Read the model definition and answer for the solid it produces. Units are mm, in the model's axes. A direction names the side the tool comes from. Round coordinates to 2 decimals unless told otherwise and drop trailing zeros. Order: outer loops, then holes, each group sorted by start corner. A loop starts at its lowest first (then second) coordinate and runs counter-clockwise, first axis right, second up. Notation, with made-up numbers: (2.5, 1) -> (14.5, 1) arc R22 cw to (14.5, 18) -> close; hole circle Ø8 at (18.25, -21). An arc over 180 degrees is marked (long way). Use a Markdown table: item, result. Add a question column.
1. Consider L1, parallel to X at y = -39.5, z = 6.25; L2, parallel to X at y = -26, z = 8.75; L3, parallel to X at y = -31.5, z = 3.5. Determine where each line is inside the solid, lowest interval first. Write a range as [from, to].
2. For faces 4 (the face through (-5, -26, 10)), 5 (the face through (-4, -46.502, 2)), 6 (the face through (66.314, -41.485, 6.302)), determine the directions among +Z, -Z, +X, -X, +Y, -Y from which every point of the face is accessible in a straight line to the end or side of a thin tool.
3. Given pin 1 (3 mm diameter, centred on y = -35, z = 4.5, fed in from -X); pin 2 (2 mm diameter, centred on x = 65.5, y = -39.5, fed in from +Z); pin 3 (5 mm diameter, centred on y = -18, z = 1.5, fed in from +X), each flat-ended and moving along its own axis, determine where each tip first touches the part or whether it passes through.
4. The mould has two halves that part along Y. Classify faces 1 (the face through (102.314, -30.797, 8.574)), 2 (the face through (-4, -26, 4)), 3 (the face through (-5.329, 1.994, 8.574)): +Y half, -Y half, draft (parallel to the pull), parting line (faces both ways), or undercut.
5. Section B-B, the plane z = 8 is taken. Give the vertices of the cut face in (x, y), then the cut area to 3 significant figures.
```python
from build123d import *

# Parameters (mm, degrees)
EXTRUDE_1_DEPTH     = 10
FILLET_1_R          = 15
FILLET_2_R          = 5
SKETCH_2_R          = 2
CUT_EXTRUDE_1_DEPTH = 7.5
SKETCH_3_W          = 46
SKETCH_3_H          = 40
CUT_EXTRUDE_2_DEPTH = 4
SKETCH_8_R          = 3
CUT_EXTRUDE_3_DEPTH = 131.716858695


with BuildPart() as part:
    # 草圖1 → 填料-伸長1 (new body)
    with BuildSketch(Plane.XY):
        Polygon((-123.946188341, 3.497757848), (-102.699073989, -56.502242152), (94.806697307, -56.502242152), (116.053811659, 3.497757848), align=None)
    extrude(amount=EXTRUDE_1_DEPTH)

    # 圓角1
    fillet_1_edges = [part.edges().sort_by_distance(p)[0] for p in [
        (116.053811659, 3.497757848, 5),
        (94.806697307, -56.502242152, 5),
        (-102.699073989, -56.502242152, 5),
        (-123.946188341, 3.497757848, 5),
    ]]
    fillet(fillet_1_edges, radius=FILLET_1_R)

    # 圓角2
    fillet_2_edges = [part.edges().sort_by_distance(p)[0] for p in [
        (107.078925905, -2.845064302, 10),
        (103.657146356, -31.509345041, 10),
        (92.862923252, -53.75186548, 10),
        (-3.946188341, -56.502242152, 10),
        (-100.755299934, -53.75186548, 10),
        (-111.549523037, -31.509345041, 10),
        (-114.971302586, -2.845064302, 10),
        (-3.946188341, 3.497757848, 10),
        (-114.971302586, -2.845064302, 0),
        (-111.549523037, -31.509345041, 0),
        (-100.755299934, -53.75186548, 0),
        (-3.946188341, -56.502242152, 0),
        (92.862923252, -53.75186548, 0),
        (103.657146356, -31.509345041, 0),
        (107.078925905, -2.845064302, 0),
        (-3.946188341, 3.497757848, 0),
    ]]
    fillet(fillet_2_edges, radius=FILLET_2_R - 0.0001)  # a hair under: the kernel refuses the full size

    # 草圖2 → 除料-伸長1 (cut)
    with BuildSketch(Plane.XY.offset(10)):
        with Locations((-73.946188341, -23.502242152)):
            Circle(SKETCH_2_R)
        with Locations((-73.946188341, -39.502242152)):
            Circle(SKETCH_2_R)
        with Locations(Location((66.053811659, -39.502242152, 0), (0, 0, 180))):
            Circle(SKETCH_2_R)
        with Locations(Location((66.053811659, -23.502242152, 0), (0, 0, 180))):
            Circle(SKETCH_2_R)
    extrude(amount=-CUT_EXTRUDE_1_DEPTH, mode=Mode.SUBTRACT)

    # 草圖3 → 除料-伸長2 (cut)
    with BuildSketch(Plane(origin=(0, 0, 0), x_dir=(-1, 0, 0), z_dir=(0, 0, -1))):
        with Locations((3.946188341, -26.502242152)):
            Rectangle(SKETCH_3_W, SKETCH_3_H)
    extrude(amount=-CUT_EXTRUDE_2_DEPTH, mode=Mode.SUBTRACT)

    # 草圖8 → 除料-伸長3 (cut, through all)
    with BuildSketch(Plane(origin=(0, 0, 4), x_dir=(-1, 0, 0), z_dir=(0, 0, -1))):
        with Locations((15.946188341, -26.502242152)):
            Circle(SKETCH_8_R)
        with Locations(Location((-8.053811659, -26.502242152, 0), (0, 0, 180))):
            Circle(SKETCH_8_R)
    extrude(amount=-CUT_EXTRUDE_3_DEPTH, mode=Mode.SUBTRACT)


solid = part.part
```
Verdict:
| question | item | result |
|---|---|---|
| 1 | L1 | x = [-108.55, -75.95], [-71.95, 64.05], [68.05, 100.66] |
| 1 | L2 | x = [-111.7, -18.9], [-12.99, 5.1], [11.01, 103.81] |
| 1 | L3 | x = [-111.31, -26.95], [19.05, 103.42] |
| 2 | face 4 | +Z, +X, -X, +Y, -Y |
| 2 | face 5 | -Z |
| 2 | face 6 | +Z |
| 3 | pin 1 | stops at x = -110.83 |
| 3 | pin 2 | stops at z = 2.5 |
| 3 | pin 3 | stops at x = 108.74 |
| 4 | face 1 | -Y half |
| 4 | face 2 | undercut |
| 4 | face 3 | +Y half |
| 5 | outline | (-115.92, -16.18) -> (-105.3, -46.18) arc R14 ccw to (-92.1, -55.5) -> (84.21, -55.5) arc R14 ccw to (97.4, -46.18) -> (108.03, -16.18) arc R14 ccw to (94.83, 2.5) -> (-102.72, 2.5) arc R14 ccw to start; hole circle Ø4 at (-73.95, -39.5); hole circle Ø4 at (-73.95, -23.5); hole circle Ø6 at (-15.95, -26.5); hole circle Ø6 at (8.05, -26.5); hole circle Ø4 at (66.05, -39.5); hole circle Ø4 at (66.05, -23.5) |
| 5 | area | 12,200 mm2 |
